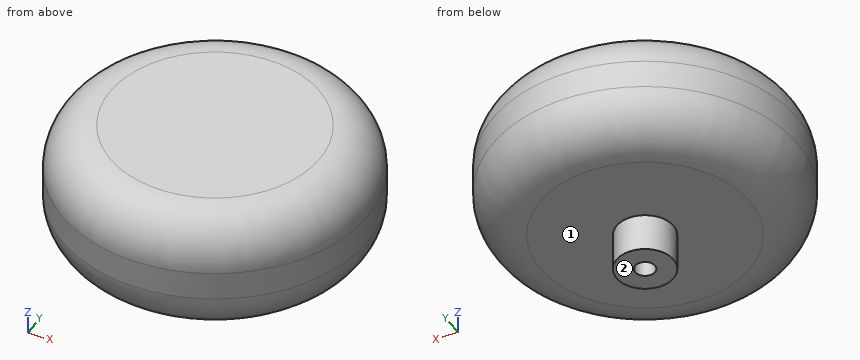
Autodesk Fusion 360 part; units mm, degrees
sketch "スケッチ1" plane through (0, 0, 0) normal (0, 0, 1) x (1, 0, 0)
  circle A0 centre (0, 0) radius 16
  dimension "d1" = 32
extrude "押し出し1" add sketch "スケッチ1" along normal blind 13
fillet "フィレット1" radius 5 2 edges at (-14.9172, -5.7858, 0) (-14.9172, -5.7858, 13)
sketch "スケッチ2" plane through (0, 0, 0) normal (0, 0, -1) x (1, 0, 0)
  circle A0 centre (0, 0) radius 11
  circle A1 centre (0, 0) radius 3
  circle A2 centre (0, 0) radius 1.05
  dimension "d6" = 6
  dimension "d7" = 2.1
extrude "押し出し2" add sketch "スケッチ2" along normal blind 4 contours A1
Input: part model. Units: mm. Frame: model coordinates. Face numbers are marked on the shaded views. A direction names the side the tool comes from. Coordinates: 2 decimals unless noted, no trailing zeros. Write each loop counter-clockwise with the first axis right and the second up, starting at its lowest first coordinate (ties: lowest second). Pieces come first, ordered by that corner, then holes. Notation, with made-up numbers: (-10.75, 16.25) - (5.25, 16.25) arc R21 cw to (5.25, 52.25) - close; hole circle Ø6 at (66.5, 74.25). An arc over 180 degrees is marked (long way). Put each result on its own line as item: value. Start each with the question number.
1) Cut plane C-C (z = 2). Return the cut outline in (x, y).
2) Cut plane A-A (x = 0). Return the cut outline in (y, z), plus the area to 3 significant figures.
3) Ray query, L1, parallel to X at y = 0, z = -1.75; L2, parallel to Z at x = 1.5, y = 8.5. Return the intervals inside material, ascending.
4) Reachability of the marked faces 1 and 2 from +Z, -Z, +X, -X, +Y, -Y: full face, straight path, thin tool, end or side. Return the list, or none.
5) Contact query for flat-ended pins moving along their axis: pin 1 (1 mm diameter, centred on x = -0.5, y = 0, fed in from -Z); pin 2 (5 mm diameter, centred on y = -6.5, z = 9, fed in from +X); pin 3 (4 mm diameter, centred on x = -8.5, y = -10, fed in from +Z); pin 4 (2 mm diameter, centred on y = 2.5, z = 5, fed in from +X). Output: stop coordinate, or through.
6) Cut plane D-D (z = 10.25). Return the cut outline in (x, y).
Resolved:
1. outline: circle Ø30 at (0, 0)
2. outline: (-16, 5) arc R5 ccw to (-11, 0) - (-3, 0) - (-3, -4) - (-1.05, -4) - (-1.05, 0) - (1.05, 0) - (1.05, -4) - (3, -4) - (3, 0) - (11, 0) arc R5 ccw to (16, 5) - (16, 8) arc R5 ccw to (11, 13) - (-11, 13) arc R5 ccw to (-16, 8) - close
2. area: 410 mm2
3. L1: x = -3 to -1.05, 1.05 to 3
3. L2: z = 0 to 13
4. face 1: -Z
4. face 2: -Z, +X, -X, +Y, -Y
5. pin 1: stops at z = 0
5. pin 2: stops at x = 15.46
5. pin 3: stops at z = 13
5. pin 4: stops at x = 15.93
6. outline: circle Ø30.93 at (0, 0)
